Autodesk Inventor part; units mm, degrees
ref_plane "YZ Plane" through (0, 0, 0) normal (1, 0, 0) x (0, 1, 0)
ref_plane "XZ Plane" through (0, 0, 0) normal (0, 1, 0) x (-1, 0, 0)
ref_plane "XY Plane" through (0, 0, 0) normal (0, 0, 1) x (1, 0, 0)
sketch "スケッチ1" plane through (0, 0, 0) normal (0, 0, 1) x (1, 0, 0)
  line L0 (-20, -2.5) -> (20, -2.5)
  line L1 (20, -2.5) -> (20, 2.5)
  line L2 (-20, 2.5) -> (-20, -2.5)
  line L3 (-20, -2.5) -> (20, 2.5) construction
  line L4 (20, -2.5) -> (-20, 2.5) construction
  line L5 (-10, 2.5) -> (10, 2.5)
  line L6 (10, 2.5) -> (10, 52.5)
  line L7 (10, 52.5) -> (-10, 52.5)
  line L8 (-10, 52.5) -> (-10, 2.5)
  line L9 (-10, 2.5) -> (10, 52.5) construction
  line L10 (10, 2.5) -> (-10, 52.5) construction
  line L11 (20, 2.5) -> (10, 2.5)
  line L12 (-10, 2.5) -> (-20, 2.5)
  line L13 (0, 52.5) -> (0, -2.5)
  point P0 (0, 0)
  point P1 (0, 27.5)
  point P2 (0, 27.5)
  point P3 (0, 0)
  dimension "d0" = 20
  dimension "d1" = 50
  dimension "d2" = 5
  dimension "d3" = 10
extrude "押し出し1" add sketch "スケッチ1" along normal mid plane 210 contours L13 L5 L11 L1 L0 | L13 L7 L6 L5
sketch "スケッチ4" plane through (0, -2.5, 105) normal (-1, 0, 0) x (0, 0, 1)
  line L0 (0, 7) -> (-33.61, 55)
  line L1 (-210, 55) -> (0, 55)
  line L2 (0, 55) -> (0, 0)
  line L3 (0, 5) -> (-210, 5)
  point P0 (-105, 2.5)
  dimension "d18" = 35
  dimension "d21" = 2
extrude "押し出し3" cut sketch "スケッチ4" against normal through all
sketch "スケッチ5" plane through (10, 2.5, -105) normal (1, 0, 0) x (0, 0, -1)
  circle A0 centre (-158, 41) radius 6.05
  line L0 (0, 0) -> (-210, 0)
  line L1 (-210, 0) -> (-210, 2)
  point P0 (-105, -2.5)
  dimension "d22" = 12.1
  dimension "d23" = 41
  dimension "d37" = 52
extrude "押し出し4" cut sketch "スケッチ5" against normal blind 10
sketch "スケッチ6" plane through (10, 2.5, 105) normal (0, 1, 0) x (1, 0, 0)
  line L0 (10, 210) -> (10, 0)
  line L1 (10, 0) -> (0, 0)
  line L2 (0, 210) -> (10, 210)
  point P0 (-10, 105)
  point P1 (5, 205)
  point P2 (5, 5)
  dimension "d27" = 5
  dimension "d28" = 5
  dimension "d29" = 5
hole "穴2" at (15, 2.5, -100) at (15, 2.5, 100) direction (0, -1, 0) diameter 3.2 end through all
sketch "スケッチ7" plane through (10, -2.5, -105) normal (-1, 0, 0) x (0, 0, 1)
  line L0 (120.4801, 39.2607) -> (161.9292, 68.2837)
  line L1 (161.9292, 68.2837) -> (180.2837, 42.0708)
  line L2 (180.2837, 42.0708) -> (138.8346, 13.0478)
  line L3 (138.8346, 13.0478) -> (120.4801, 39.2607)
  line L4 (120.4801, 39.2607) -> (180.2837, 42.0708) construction
  line L5 (161.9292, 68.2837) -> (138.8346, 13.0478) construction
  circle A0 centre (158, 46) radius 6.05
  line L6 (0, 0) -> (210, 0)
  point P0 (105, 2.5)
  dimension "d38" = 32
  dimension "d39" = 50.6
  dimension "d40" = 16
  dimension "d41" = 16
  dimension "d42" = 35
hole "穴3" at (10, 10.5478, 33.8346) at (10, 36.7607, 15.4801) at (10, 39.5708, 75.2837) direction (-1, 0, 0) diameter 4.3 end through all counterbore diameter 8 counterbore depth 5
equation "\"d40\" = 0.5 * d38"
properties part number "s_base4"
CAD build for the part. Positions are in the model's coordinates, mm. A direction names the side the tool comes from. Round coordinates to 2 decimals unless told otherwise and drop trailing zeros. Order: outer loops, then holes, each group sorted by start corner. A loop starts at its lowest first (then second) coordinate and runs counter-clockwise, first axis right, second up. Notation, with made-up numbers: (-10, 55.25) - (43, 55.25) arc R30 cw to (43, 82.25) - close; hole circle Ø10 at (47, 7.5). An arc over 180 degrees is marked (long way). Answer as CSV lines item,"result". Start each with the question number.
1. Pin check, flat tips, straight feed: pin 1 (7 mm diameter, centred on y = 36.76, z = 15.48, fed in from +X); pin 2 (6 mm diameter, centred on x = 10, y = 43.5, fed in from +Z); pin 3 (6.5 mm diameter, centred on y = 38, z = 16, fed in from +X); pin 4 (9.5 mm diameter, centred on y = 43.5, z = 53, fed in from +X). Stop position of each tip, or through.
2. Pull direction Z, two halves, no side cores. Call faces 4 (the face through (4.93, 28.164, 88.43)), 5 (the face through (5, 25, -105)), 6 (the face through (2.465, 10.453, 35.983)), 7 (the face through (15, 2.5, -1)): +Z half, -Z half, draft (parallel to the pull), parting line (faces both ways), or undercut.
3. Saw through at C-C, the plane y = 29.5. Write the cut outline in (x, z), and give its area (3 significant figures).
4. Saw through at B-B, the plane z = 5. Write the cut outline in (x, y).
5. Tool access for faces 1 (the face through (5.07, 49.5, 53.79)), 2 (the face through (5, 12, 32)), 3 (the face through (10, 27, -1)): list every direction of +Z, -Z, +X, -X, +Y, -Y with a clear straight run to the whole face (end or side of a thin tool).
6. Drill centre lines: L1, parallel to Y at x = 6, z = 53; L2, parallel to X at y = 30.5, z = -15.5; L3, parallel to Y at x = 17.5, z = -27. Where is each one in solid material? Low to high. Write a range as [from, to].
7. Saw through at D-D, the plane z = 89. Write the cut outline in (x, y).
8. Saw through at A-A, the plane z = 53. Write the cut outline in (x, y), and give its area (3 significant figures).
Model answer:
1,pin 1,"stops at x = 5"
1,pin 2,"stops at z = 79.79"
1,pin 3,"stops at x = 10"
1,pin 4,"passes through"
2,face 4,"+Z half"
2,face 5,"-Z half"
2,face 6,"undercut"
2,face 7,"draft"
3,outline,"(0, -105) - (10, -105) - (10, 87.49) - (0, 87.49) - close"
3,area,"1,920 mm²"
4,outline,"(0, -2.5) - (20, -2.5) - (20, 2.5) - (10, 2.5) - (10, 52.5) - (0, 52.5) - close"
5,face 1,"+X, -X"
5,face 2,"+X"
5,face 3,"+Z, -Z, +X, +Y"
6,L1,"y = [-2.5, 37.45], [49.55, 52.5]"
6,L2,"x = [0, 10]"
6,L3,"y = [-2.5, 2.5]"
7,outline,"(0, -2.5) - (20, -2.5) - (20, 2.5) - (10, 2.5) - (10, 27.35) - (0, 27.35) - close"
8,outline,"(0, -2.5) - (20, -2.5) - (20, 2.5) - (10, 2.5) - (10, 37.45) - (0, 37.45) - close; (0, 49.55) - (10, 49.55) - (10, 52.5) - (0, 52.5) - close"
8,area,"479 mm²"
